Here's how the part is built. I have some questions about the finished solid (model axes, mm). Give positions to 0.01 mm unless a question says otherwise; leave off trailing zeros. Loops run counter-clockwise (first coordinate to the right, second up) from the corner with the lowest first, then second, coordinate; pieces in that order, holes last. Notation, with made-up numbers: (27, 51) - (40, 51) arc R12 cw to (40, 61) - close; hole circle Ø11 at (56.25, 7.25). An arc over 180 degrees is marked (long way). Put each result on its own line as item: value. Start each with the question number.
from build123d import *

# Parameters (mm, degrees)
F0_R     = 2
F1_DEPTH = 2


# Not quite as in the source:
# - ends of sketch curves that miss each other by under 0.0002 mm in the source are joined


with BuildPart() as f1:
    # F0 (on Top) → F1 (new body)
    with BuildSketch(Plane.XY):
        with BuildLine():
            ThreePointArc((91.5, -21.3966), (91.2197291677, -20.1304747082), (90.4312844969, -19.1009214093))
            Line((90.4312844969, -19.1009214093), (29.337212, 32.295678))
            ThreePointArc((29.337212, 32.295678), (28.4337805172, 32.818424586), (27.405927, 33))
            Line((27.405927, 33), (-75.25736, 33))
            ThreePointArc((-75.25736, 33), (-76.4054102971, 32.7716385975), (-77.3786803436, 32.1213203436))
            Line((-77.3786803436, 32.1213203436), (-90.621321, 18.87868))
            ThreePointArc((-90.621321, 18.87868), (-91.2716385975, 17.9054092971), (-91.5, 16.757359))
            Line((-91.5, 16.757359), (-91.5, -30))
            ThreePointArc((-91.5, -30), (-90.6213203436, -32.1213203436), (-88.5, -33))
            Line((-88.5, -33), (88.5, -33))
            ThreePointArc((88.5, -33), (90.6213203436, -32.1213203436), (91.5, -30))
            Line((91.5, -30), (91.5, -21.3966))
        make_face()
        with Locations((-84.7, -27)):
            Circle(F0_R, mode=Mode.SUBTRACT)
        with Locations((84.5, -27)):
            Circle(F0_R, mode=Mode.SUBTRACT)
        with Locations((-84.7, 11.8)):
            Circle(F0_R, mode=Mode.SUBTRACT)
        with Locations((-70.5, 26.1)):
            Circle(F0_R, mode=Mode.SUBTRACT)
        with Locations((22, 26.1)):
            Circle(F0_R, mode=Mode.SUBTRACT)
    extrude(amount=F1_DEPTH)


solid = f1.part
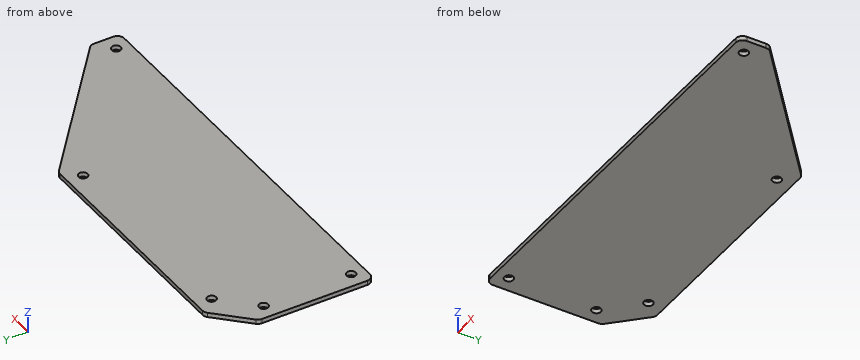
1) Suppose I cut it at B-B on z = 0.7. Please give me the cut outline in (x, y), plus the area to 3 significant figures.
2) Suppose I cut it at A-A on x = -70.5. Please give me the cut outline in (y, z).
3) Suppose I cut it at C-C on y = 11.8. Please give me the cut outline in (x, z), plus the area to 3 significant figures.
4) Suppose I cut it at D-D on y = -27. Please give me the cut outline in (x, z).
5) I need wall thicknesses on line 1 (Y direction, x = 22, z = 0.7); line 2 (X direction, y = 11, z = 1.2); line 3 (X direction, y = 13, z = 0.7). Which ranges of each line are inside material? Lowest first, please.
6) I'm going to push flat-ended pins straight in: P1, Ø6.5, axis at x = -84.7, y = -27, coming from the +Z side; P2, Ø1, axis at y = -8, z = 1, coming from the +X side. Where does each tip first touch, or does it pass through?
Ans:
1. outline: (-91.5, -30) arc R3 ccw to (-88.5, -33) - (88.5, -33) arc R3 ccw to (91.5, -30) - (91.5, -21.4) arc R3 ccw to (90.43, -19.1) - (29.34, 32.3) arc R3 ccw to (27.41, 33) - (-75.26, 33) arc R3 ccw to (-77.38, 32.12) - (-90.62, 18.88) arc R3 ccw to (-91.5, 16.76) - close; hole circle Ø4 at (-84.7, -27); hole circle Ø4 at (-84.7, 11.8); hole circle Ø4 at (-70.5, 26.1); hole circle Ø4 at (22, 26.1); hole circle Ø4 at (84.5, -27)
1. area: 10,200 mm²
2. outline: (-33, 0) - (24.1, 0) - (24.1, 2) - (-33, 2) - close; (28.1, 0) - (33, 0) - (33, 2) - (28.1, 2) - close
3. outline: (-91.5, 0) - (-86.7, 0) - (-86.7, 2) - (-91.5, 2) - close; (-82.7, 0) - (53.7, 0) - (53.7, 2) - (-82.7, 2) - close
3. area: 282 mm²
4. outline: (-91.5, 0) - (-86.7, 0) - (-86.7, 2) - (-91.5, 2) - close; (-82.7, 0) - (82.5, 0) - (82.5, 2) - (-82.7, 2) - close; (86.5, 0) - (91.5, 0) - (91.5, 2) - (86.5, 2) - close
5. line 1: y = -33 to 24.1, 28.1 to 33
5. line 2: x = -91.5 to -86.53, -82.87 to 54.65
5. line 3: x = -91.5 to -86.3, -83.1 to 52.27
6. P1: stops at z = 2
6. P2: stops at x = 77.83
